Build history of the part. All positions in model axes, mm. Face numbers are marked on the shaded views. Coordinates: 2 decimals unless noted, no trailing zeros. Loops run counter-clockwise (first coordinate to the right, second up) from the corner with the lowest first, then second, coordinate; pieces in that order, holes last. Notation, with made-up numbers: (80, 61) - (95, 61) arc R22 cw to (95, 85) - close; hole circle Ø11 at (63.5, 38.5). An arc over 180 degrees is marked (long way). One line per item, written item: value.
```python
from build123d import *

# Parameters (mm, degrees)
SKETCH1_R           = 10
BOSS_EXTRUDE2_DEPTH = 79
SKETCH5_R           = 12.5
BOSS_EXTRUDE3_DEPTH = 2
SKETCH6_R           = 12.5
BOSS_EXTRUDE4_DEPTH = 2
BOSS_EXTRUDE4_TAPER = 80
SKETCH7_R           = 8
CUT_EXTRUDE1_DEPTH  = 79


with BuildPart() as part:
    # Sketch1 → Boss-Extrude2 (new body)
    with BuildSketch(Plane.XY):
        Circle(SKETCH1_R)
    extrude(amount=-BOSS_EXTRUDE2_DEPTH)

    # Sketch5 → Boss-Extrude3 (add)
    with BuildSketch(Plane.XY):
        Circle(SKETCH5_R)
    extrude(amount=BOSS_EXTRUDE3_DEPTH)

    # Sketch6 → Boss-Extrude4 (add)
    with BuildSketch(Plane.XY.offset(2)):
        Circle(SKETCH6_R)
    extrude(amount=BOSS_EXTRUDE4_DEPTH, taper=BOSS_EXTRUDE4_TAPER)

    # Sketch7 → Cut-Extrude1 (cut)
    with BuildSketch(Plane(origin=(0, 0, -79), x_dir=(-1, 0, 0), z_dir=(0, 0, -1))):
        Circle(SKETCH7_R)
    extrude(amount=-CUT_EXTRUDE1_DEPTH, mode=Mode.SUBTRACT)


solid = part.part
```
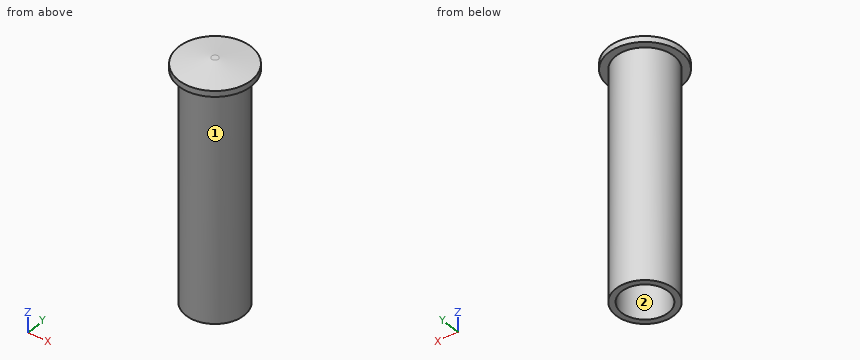
Item 1: Drop flat-ended pins along their axis: P1, Ø1.5, axis at x = -1, y = 4, coming from the -Z side; P2, Ø1, axis at x = 6, z = -30, coming from the -Y side; P3, Ø3, axis at x = -4.5, z = -24, coming from the +Y side. Give the stop position or say it passes through.
Check result:
P1: stops at z = 0
P2: stops at y = -8.35
P3: stops at y = 9.54
Item 2: Probe probe 1 along X at (y, z) = (-0.25, -31.5); probe 2 along X at (y, z) = (-4, -60.5). List the from-to ranges inside material, lowest first. Write a range as from..to.
Check result:
probe 1: x = -10..-8, 8..10
probe 2: x = -9.17..-6.93, 6.93..9.17
Item 3: Cut at A-A, the plane x = 0. Write the cut outline in (y, z).
Check result:
outline: (-12.5, 0) - (-10, 0) - (-10, -79) - (-8, -79) - (-8, 0) - (8, 0) - (8, -79) - (10, -79) - (10, 0) - (12.5, 0) - (12.5, 2) - (1.16, 4) - (-1.16, 4) - (-12.5, 2) - close
Item 4: Cut at C-C, the plane z = -71. Write the cut outline in (x, y), then the cut area to 3 significant figures.
Check result:
outline: circle Ø20 at (0, 0); hole circle Ø16 at (0, 0)
area: 113 mm^2
Item 5: Pull direction X, two halves, no side cores. Call the marked faces 1 and 2: released by +X, released by -X, zero draft, split by the parting line, or undercut.
Check result:
face 1: split by the parting line
face 2: undercut
